Work out the finished part from the listing and answer in its coordinate system (mm). Face numbers are marked on the shaded views. A direction names the side the tool comes from. Coordinates: 2 decimals unless noted, no trailing zeros. Write each loop counter-clockwise with the first axis right and the second up, starting at its lowest first coordinate (ties: lowest second). Pieces come first, ordered by that corner, then holes. Notation, with made-up numbers: (52, -23) - (103, -23) arc R21 cw to (103, -13) - close; hole circle Ø7 at (53.25, -8). An arc over 180 degrees is marked (long way). Use a Markdown table: item, result. Add a question column.
(1) The part is cut by section D-D, the plane x = 9.5. Give the vertices of the cut face in (y, z).
(2) A tool of negligible diameter and unlimited length cuts with its end or side. For the marked faces 5, 6 and 7, from which of +Z, -Z, +X, -X, +Y, -Y can it reach the whole face along a straight path? Write none if from no direction.
(3) For a pull along Y with two mould halves and no side action, classify the marked faces 1, 2, 3 and 4 as released by +Y, released by -Y, zero draft, split by the parting line, or undercut.
(4) The part is cut by section A-A, the plane z = 5.5. Give the vertices of the cut face in (x, y), then the cut area to 3 significant figures.
(5) Given pin 1 Ø1.6 at (x, y) = (4, -47) entering from -Z; pin 2 Ø5.5 at (x, z) = (6.5, 3.5) entering from +Y; pin 3 Ø3 at (x, y) = (5.5, -18.5) entering from +Z; pin 4 Ø5 at (x, y) = (7.5, -38.5) entering from -Z, each flat-ended and moving along its own axis, determine where each tip first touches the part or whether it passes through.
(6) Find the intervals of material crossed by line 1 (Y direction, x = 2, z = 5); line 2 (Z direction, x = 6, y = -25); line 3 (Z direction, x = 5.75, y = -24.5), in increasing order. Write a range as from..to.
(7) The part is cut by section B-B, the plane x = 7.5. Give the vertices of the cut face in (y, z), then the cut area to 3 significant figures.
(8) The part is cut by section C-C, the plane x = 4.75. State how many separate pieces and enclosed holes the cut face has, then the cut area to 3 significant figures.
from build123d import *

# Parameters (mm, degrees)
SKETCH1_W           = 10
SKETCH1_H           = 50
BOSS_EXTRUDE1_DEPTH = 40
CUT_EXTRUDE1_DEPTH  = 40
CUT_EXTRUDE2_DEPTH  = 40
SKETCH4_W           = 10
SKETCH4_H           = 7
SKETCH4_H_2         = 12
CUT_EXTRUDE3_DEPTH  = 6
SKETCH5_R           = 1.5
CUT_EXTRUDE4_DEPTH  = 38
CUT_EXTRUDE5_DEPTH  = 38
FILLET1_R           = 1.5


with BuildPart() as part:
    # Sketch1 → Boss-Extrude1 (new body)
    with BuildSketch(Plane.XY):
        with Locations((5, -25)):
            Rectangle(SKETCH1_W, SKETCH1_H)
    extrude(amount=BOSS_EXTRUDE1_DEPTH)

    # Sketch2 → Cut-Extrude1 (cut)
    with BuildSketch(Plane(origin=(10, 0, 0), x_dir=(0, 0, -1), z_dir=(1, 0, 0))):
        Polygon((-27.429786362, -11.848127256), (0, 0), (-40, 0), (-40, -17.277753606), align=None)
        Polygon((-23.790339217, -37.357038236), (-40, -17.277753606), (-40, -50), (-13.583893856, -50), align=None)
    extrude(amount=-CUT_EXTRUDE1_DEPTH, mode=Mode.SUBTRACT)

    # Sketch3 → Cut-Extrude2 (cut)
    with BuildSketch(Plane(origin=(10, 0, 0), x_dir=(0, 0, -1), z_dir=(1, 0, 0))):
        Polygon((-30.211268677, -13.049571408), (-21.196168582, -40.570497868), (-40, -17.277753606), align=None)
    extrude(amount=-CUT_EXTRUDE2_DEPTH, mode=Mode.SUBTRACT)

    # Sketch4 → Cut-Extrude3 (cut)
    with BuildSketch(Plane(origin=(0, 0, 0), x_dir=(-1, 0, 0), z_dir=(0, 0, -1))):
        with Locations((-5, -3.5)):
            Rectangle(SKETCH4_W, SKETCH4_H)
        with Locations((-5, -17)):
            Rectangle(SKETCH4_W, SKETCH4_H_2)
        with Locations((-5, -33)):
            Rectangle(SKETCH4_W, SKETCH4_H_2)
        with Locations((-5, -46.5)):
            Rectangle(SKETCH4_W, SKETCH4_H)
    extrude(amount=-CUT_EXTRUDE3_DEPTH, mode=Mode.SUBTRACT)

    # Sketch5 → Cut-Extrude4 (cut)
    with BuildSketch(Plane.XZ.offset(43)):
        with Locations((5.065925619, 2.867770419)):
            Circle(SKETCH5_R)
    extrude(amount=-CUT_EXTRUDE4_DEPTH, mode=Mode.SUBTRACT)

    # Sketch6 → Cut-Extrude5 (cut)
    with BuildSketch(Plane.XZ.offset(43)):
        with BuildLine():
            ThreePointArc((10, 2.741877925), (4.957177855, 0.700758069), (0, 2.941876799))
            Line((0, 2.941876799), (0, 0))
            Line((0, 0), (10, 0))
            Line((10, 0), (10, 2.741877925))
        make_face()
    extrude(amount=-CUT_EXTRUDE5_DEPTH, mode=Mode.SUBTRACT)

    # Fillet1
    fillet1_edges = [part.edges().sort_by_distance(p)[0] for p in [
        (0, -7.820617225, 18.105634338),
        (5, -2.591663041, 6),
        (10, -7.820617225, 18.105634338),
        (0, -50, 9.791946928),
        (10, -50, 9.791946928),
        (5, -50, 6),
        (10, -45.285248934, 17.390031219),
        (5, -50, 13.583893856),
        (0, -45.285248934, 17.390031219),
        (0, -26.810034638, 25.703718629),
        (5, -13.049571408, 30.211268677),
        (10, -26.810034638, 25.703718629),
        (5, -40.570497868, 21.196168582),
        (0, -46.5, 6),
        (0, -33, 6),
        (0, -17, 6),
        (10, -46.5, 6),
        (10, -33, 6),
        (10, -17, 6),
    ]]
    fillet(fillet1_edges, radius=FILLET1_R)


solid = part.part
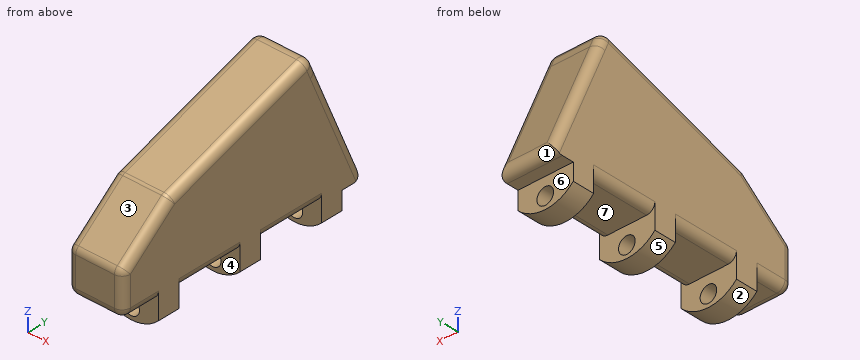
Model answer:
| question | item | result |
|---|---|---|
| 1 | outline | (-49.62, 7.5) arc R1.12 ccw to (-48.5, 6.38) - (-43, 6.38) - (-43, 2.29) - (-39, 2.29) - (-39, 6.38) - (-27, 6.38) - (-27, 2.29) - (-23, 2.29) - (-23, 6.38) - (-11, 6.38) - (-11, 2.29) - (-7, 2.29) - (-7, 6) - (-4.87, 6) arc R1.5 ccw to (-3.45, 7.03) - (-12.86, 28.8) arc R1.12 ccw to (-14.23, 29.42) - (-40.19, 20.92) arc R1.12 ccw to (-40.54, 20.73) - (-49.2, 13.74) arc R1.12 ccw to (-49.62, 12.87) - close |
| 2 | face 5 | -Z, +Y, -Y |
| 2 | face 6 | -Z, +X, -X, +Y |
| 2 | face 7 | -Z, +X, -X |
| 3 | face 1 | released by +Y |
| 3 | face 2 | zero draft |
| 3 | face 3 | released by -Y |
| 3 | face 4 | undercut |
| 4 | outline | (0, -43) - (10, -43) - (10, -39) - (0, -39) - close; (0, -27) - (10, -27) - (10, -23) - (0, -23) - close; (0, -11) - (10, -11) - (10, -7) - (0, -7) - close |
| 4 | area | 120 mm^2 |
| 5 | pin 1 | z = 6 |
| 5 | pin 2 | y = -4.04 |
| 5 | pin 3 | z = 28.92 |
| 5 | pin 4 | z = 0.7 |
| 6 | line 1 | -43..-39, -27..-23, -11..-7 |
| 6 | line 2 | 0.76..1.69, 4.04..26.3 |
| 6 | line 3 | 0.73..1.53, 4.2..26.46 |
| 7 | outline | (-50, 7.5) arc R1.5 ccw to (-48.5, 6) - (-43, 6) - (-43, 1.13) - (-39, 1.13) - (-39, 6) - (-27, 6) - (-27, 1.13) - (-23, 1.13) - (-23, 6) - (-11, 6) - (-11, 1.13) - (-7, 1.13) - (-7, 6) - (-4.87, 6) arc R1.5 ccw to (-3.5, 8.09) - (-12.51, 28.95) arc R1.5 ccw to (-14.35, 29.79) - (-40.31, 21.28) arc R1.5 ccw to (-40.78, 21.02) - (-49.44, 14.03) arc R1.5 ccw to (-50, 12.87) - close |
| 7 | area | 833 mm^2 |
| 8 | separate pieces | 4 |
| 8 | enclosed holes | 0 |
| 8 | area | 802 mm^2 |
